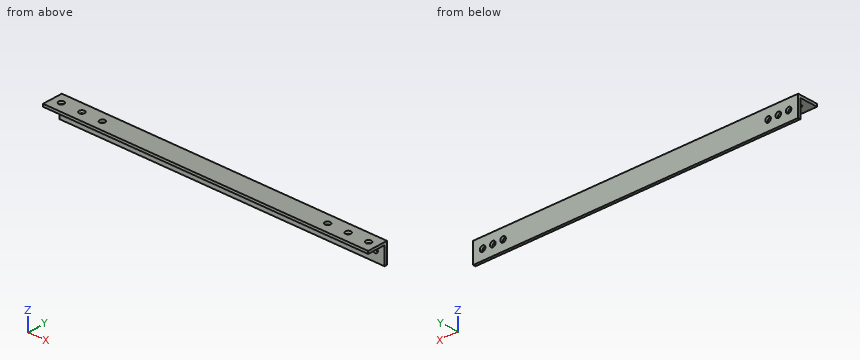
```python
from build123d import *

# Parameters (mm, degrees)
BOSS_EXTRUDE1_DEPTH = 403.225
SKETCH2_R           = 3.429
CUT_EXTRUDE1_DEPTH  = 3.175
SKETCH3_R           = 3.429
CUT_EXTRUDE2_DEPTH  = 3.175


with BuildPart() as part:
    # Sketch1 → Boss-Extrude1 (new body)
    with BuildSketch(Plane(origin=(0, 0, 0), x_dir=(0, 0, -1), z_dir=(1, 0, 0))):
        Polygon((0, 0), (25.4, 0), (25.4, -3.175), (3.175, -3.175), (3.175, -25.4), (0, -25.4), align=None)
    extrude(amount=BOSS_EXTRUDE1_DEPTH)

    # Sketch2 → Cut-Extrude1 (cut)
    with BuildSketch(Plane.XY):
        with Locations((11.1125, -12.7)):
            Circle(SKETCH2_R)
        with Locations((36.5125, -12.7)):
            Circle(SKETCH2_R)
        with Locations((61.9125, -12.7)):
            Circle(SKETCH2_R)
        with Locations((341.3125, -12.7)):
            Circle(SKETCH2_R)
        with Locations((366.7125, -12.7)):
            Circle(SKETCH2_R)
        with Locations((392.1125, -12.7)):
            Circle(SKETCH2_R)
    extrude(amount=-CUT_EXTRUDE1_DEPTH, mode=Mode.SUBTRACT)

    # Sketch3 → Cut-Extrude2 (cut)
    with BuildSketch(Plane(origin=(0, 0, 0), x_dir=(1, 0, 0), z_dir=(0, 1, 0))):
        with Locations((11.8999, 12.7)):
            Circle(SKETCH3_R)
        with Locations((24.5999, 12.7)):
            Circle(SKETCH3_R)
        with Locations((37.2999, 12.7)):
            Circle(SKETCH3_R)
        with Locations((365.9251, 12.7)):
            Circle(SKETCH3_R)
        with Locations((378.6251, 12.7)):
            Circle(SKETCH3_R)
        with Locations((391.3251, 12.7)):
            Circle(SKETCH3_R)
    extrude(amount=-CUT_EXTRUDE2_DEPTH, mode=Mode.SUBTRACT)


solid = part.part
```
Here's how the part is built. I have some questions about the finished solid (model axes, mm). Give positions to 0.01 mm unless a question says otherwise; leave off trailing zeros. Order: outer loops, then holes, each group sorted by start corner. A loop starts at its lowest first (then second) coordinate and runs counter-clockwise, first axis right, second up. Notation, with made-up numbers: M 54,79.5 L 62,79.5 A25 cw 62,112.5 Z; hole C -18,10 d4. An arc over 180 degrees is marked long. Use a Markdown table: item, result. Add a question column.
1. For pin 1 Ø1 at (y, z) = (-3.5, -9.5) entering from +X (3 decimals); pin 2 Ø6 at (x, z) = (214.5, -7.5) entering from -Y (3 decimals); pin 3 Ø11 at (x, y) = (249.5, -13.5) entering from -Z (3 decimals); pin 4 Ø6 at (x, z) = (24.6, -12.7) entering from -Y, each with a flat end and sliding along its axis, tell me the tip position at first contact or that it passes through.
2. Suppose I cut it at C-C (x = 296). List the corners of the cut face in (y, z) for me (3 decimals), and give its area (3 significant figures).
3. Suppose I cut it at B-B (y = -12.7). List the corners of the cut face in (x, z) for me (1 decimal), and give its area (3 significant figures).
4. I need wall thicknesses on probe 1 along Y at (x, z) = (61.5, -2.25); probe 2 along Z at (x, y) = (373.5, -9.75) (3 decimals). Which ranges of each line are inside material? Lowest first, please. Write a range as from..to.
5. Suppose I cut it at A-A (z = -12.7). List the corners of the cut face in (x, y) for me (3 decimals).
Results list:
| question | item | result |
|---|---|---|
| 1 | pin 1 | stops at x = 403.225 |
| 1 | pin 2 | stops at y = -3.175 |
| 1 | pin 3 | stops at z = -3.175 |
| 1 | pin 4 | passes through |
| 2 | outline | M -25.4,-3.175 L -3.175,-3.175 L -3.175,-25.4 L 0,-25.4 L 0,0 L -25.4,0 Z |
| 2 | area | 151 mm² |
| 3 | outline | M 0,-3.2 L 7.7,-3.2 L 7.7,0 L 0,0 Z; M 14.5,-3.2 L 33.1,-3.2 L 33.1,0 L 14.5,0 Z; M 39.9,-3.2 L 58.5,-3.2 L 58.5,0 L 39.9,0 Z; M 65.3,-3.2 L 337.9,-3.2 L 337.9,0 L 65.3,0 Z; M 344.7,-3.2 L 363.3,-3.2 L 363.3,0 L 344.7,0 Z; M 370.1,-3.2 L 388.7,-3.2 L 388.7,0 L 370.1,0 Z; M 395.5,-3.2 L 403.2,-3.2 L 403.2,0 L 395.5,0 Z |
| 3 | area | 1,150 mm² |
| 4 | probe 1 | y = -25.4..-16.1, -9.3..0 |
| 4 | probe 2 | z = -3.175..0 |
| 5 | outline | M 0,-3.175 L 8.471,-3.175 L 8.471,0 L 0,0 Z; M 15.329,-3.175 L 21.171,-3.175 L 21.171,0 L 15.329,0 Z; M 28.029,-3.175 L 33.871,-3.175 L 33.871,0 L 28.029,0 Z; M 40.729,-3.175 L 362.496,-3.175 L 362.496,0 L 40.729,0 Z; M 369.354,-3.175 L 375.196,-3.175 L 375.196,0 L 369.354,0 Z; M 382.054,-3.175 L 387.896,-3.175 L 387.896,0 L 382.054,0 Z; M 394.754,-3.175 L 403.225,-3.175 L 403.225,0 L 394.754,0 Z |
